The listing builds one solid part. Answer for the finished solid, in the listing's coordinates (mm). Give positions to 0.01 mm unless a question says otherwise; leave off trailing zeros. Loops run counter-clockwise (first coordinate to the right, second up) from the corner with the lowest first, then second, coordinate; pieces in that order, holes last. Notation, with made-up numbers: (-34.5, -22.5) - (19.5, -22.5) arc R10 cw to (19.5, -3.5) - close; hole circle Ø2 at (6, 15.25). An arc over 180 degrees is marked (long way). Write item = value, one per line. Start each with the question number.
1) The part is cut by section B-B on x = 0.6. Write down the section's boundary in (y, z), plus the area to 3 significant figures.
2) The part is cut by section A-A on z = -16. Write down the section's boundary in (x, y).
3) Consider probe 1 along Y at (x, z) = (1.5, -16.5); probe 2 along Y at (x, z) = (0.15, 24); probe 3 along Y at (x, z) = (0.6, 10). Determine where each line is inside the solid, lowest interval first.
4) The part is cut by section D-D on z = 22. Write down the section's boundary in (x, y), plus the area to 3 significant figures.
5) The part is cut by section C-C on y = -19.5. Write down the section's boundary in (x, z).
Autodesk Inventor part; units mm, degrees
ref_plane "YZ Plane" through (0, 0, 0) normal (1, 0, 0) x (0, 1, 0)
ref_plane "XZ Plane" through (0, 0, 0) normal (0, 1, 0) x (-1, 0, 0)
ref_plane "XY Plane" through (0, 0, 0) normal (0, 0, 1) x (1, 0, 0)
sketch "Sketch1" plane through (0, 0, 0) normal (1, 0, 0) x (0, 1, 0)
  circle A0 centre (1.8217, 14.5615) radius 2.1844
  circle A1 centre (16.7653, 25.7818) radius 2.1844
  circle A2 centre (16.7653, 0.3818) radius 2.1844
  circle A3 centre (19.1795, -17.4456) radius 2.1844
  circle A4 centre (-18.0648, -25.4753) radius 2.1844
  circle A5 centre (19.1795, -17.4456) radius 6.35
  circle A6 centre (16.7653, 25.7818) radius 6.35
  circle A7 centre (-18.0648, -25.4753) radius 6.35
  line L0 (20.6395, -23.6254) -> (-16.7263, -31.6826)
  line L1 (25.5295, -17.4456) -> (23.1153, 25.7818)
  line L2 (14.5809, 31.7443) -> (-6.9779, 18.5698)
  line L3 (-8.2796, 17.0161) -> (-23.9793, -23.1643)
  arc A8 (-6.9779, 18.5698) -> (-8.2796, 17.0161) centre (-5.3223, 15.8607) ccw
  point P0 (0, 0)
  dimension "d0" = 12.7
  dimension "d1" = 12.7
  dimension "d2" = 12.7
  dimension "d3" = 3.175
extrude "Extrusion1" add sketch "Sketch1" along normal blind 1.5875 contours A5 L1 | L0 A7 L3 A8 L2 A6 L1 A5 | A7 | A6 L2 picked at (18.545, -22.3352) picked at (14.1871, 29.9232)
properties part number "lbsupport"
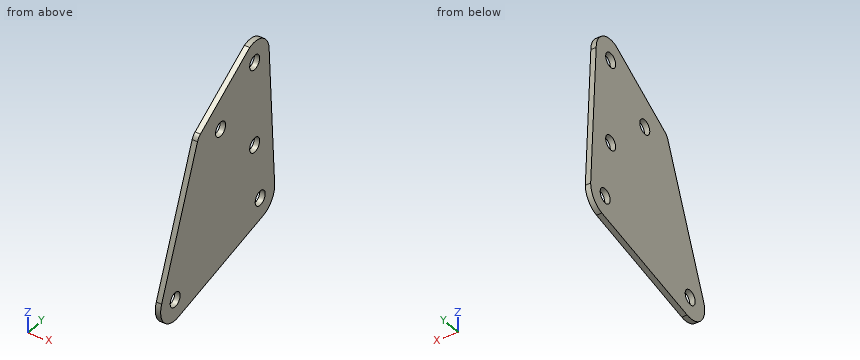
Answer below:
q1.outline = (-23.98, -23.16) arc R6.35 ccw to (-16.73, -31.68) - (20.64, -23.63) arc R6.35 ccw to (25.53, -17.45) - (23.12, 25.78) arc R6.35 ccw to (14.58, 31.74) - (-6.98, 18.57) arc R3.18 ccw to (-8.28, 17.02) - close; hole circle Ø4.37 at (-18.06, -25.48); hole circle Ø4.37 at (1.82, 14.56); hole circle Ø4.37 at (16.77, 0.38); hole circle Ø4.37 at (16.77, 25.78); hole circle Ø4.37 at (19.18, -17.45)
q1.area = 2,080 mm2
q2.outline = (0, -21.18) - (1.59, -21.18) - (1.59, 17.54) - (0, 17.54) - close; (0, 20.82) - (1.59, 20.82) - (1.59, 25.45) - (0, 25.45) - close
q3.probe_1 = -21.38 to 17.21, 21.15 to 25.48
q3.probe_2 = 1.91 to 15.5, 18.03 to 23.21
q3.probe_3 = -11.02 to 24
q4.outline = (0, -1.36) - (1.59, -1.36) - (1.59, 23.33) - (0, 23.33) - close
q4.area = 39.2 mm2
q5.outline = (0, -31.66) - (1.59, -31.66) - (1.59, -27.12) - (0, -27.12) - close; (0, -23.83) - (1.59, -23.83) - (1.59, -11.7) - (0, -11.7) - close
